Autodesk Inventor part; units mm, degrees
ref_plane "b1_XY" through (0, 7.8994, 0) normal (1, 0, 0) x (0, 0, -1)
ref_plane "b1_YZ" through (0, 7.8994, 0) normal (0, 0, -1) x (0, 1, 0)
ref_plane "b1_ZX" through (0, 7.8994, 0) normal (0, 1, 0) x (1, 0, 0)
sketch "Sketch_1" plane through (0, 0, 0) normal (0, 0, 1) x (1, 0, 0)
  line L0 (18.1102, 0) -> (0, 0)
  line L1 (0, 0) -> (0, 10.8585)
  line L2 (0, 10.8585) -> (18.1102, 10.8585)
  line L3 (18.1102, 10.8585) -> (18.1102, 0)
  line L4 (18.1102, 0) -> (0, 0)
revolve "Revolution1" add sketch "Sketch_1" angle 360 about axis through (18.1102, 0, 0) along (1, 0, 0)
sketch "Sketch_2" plane through (0, 0, 0) normal (0, 0, 1) x (1, 0, 0)
  line L0 (0, 0) -> (-12.7508, 0)
  line L1 (-12.7508, 0) -> (-12.7508, 7.098)
  line L2 (-12.7508, 7.098) -> (-11.9113, 7.9375)
  line L3 (-11.9113, 7.9375) -> (0, 7.9375)
  line L4 (0, 7.9375) -> (0, 0)
  line L5 (0, 0) -> (-12.7508, 0)
revolve "Revolution2" add sketch "Sketch_2" angle 360 about axis through (0, 0, 0) along (1, 0, 0)
thread "Thread1"
sketch "Sketch_6" plane through (0, 0, 0) normal (0, 0, 1) x (1, 0, 0)
  line L0 (27.7622, 0) -> (18.1102, 0)
  line L1 (18.1102, 0) -> (18.1102, 10.3505)
  line L2 (18.1102, 10.3505) -> (21.4122, 10.3505)
  line L3 (21.4122, 10.3505) -> (21.4122, 8.9027)
  line L4 (21.4122, 8.9027) -> (22.3266, 8.9027)
  line L5 (22.3266, 8.9027) -> (23.0505, 9.6266)
  line L6 (23.0505, 9.6266) -> (27.0002, 9.6266)
  line L7 (27.0002, 9.6266) -> (27.7622, 8.8646)
  line L8 (27.7622, 8.8646) -> (27.7622, 0)
  line L9 (27.7622, 0) -> (18.1102, 0)
revolve "Revolution3" add sketch "Sketch_6" angle 360 about axis through (27.7622, 0, 0) along (1, 0, 0)
sketch "Sketch_7" plane through (0, 0, 0) normal (1, 0, 0) x (0, 1, 0)
  circle A0 centre (0, 0) radius 3.175
extrude "Extrusion1" cut sketch "Sketch_7" along normal mid plane 111.0488
sketch "Sketch_8" plane through (11.8872, 0, 0) normal (0, 0, 1) x (0, -1, 0)
  line L0 (0, 0) -> (-11.7085, 0)
  line L1 (-11.7085, 0) -> (-11.7085, 6.4547)
  line L2 (-11.7085, 6.4547) -> (-10.0692, 4.8153)
  line L3 (-10.0692, 4.8153) -> (0, 4.501)
  line L4 (0, 4.501) -> (0, 0)
  line L5 (0, 0) -> (-11.7085, 0)
revolve "Revolution4" cut sketch "Sketch_8" angle 360 about axis through (11.8872, 0, 0) along (0, -1, 0)
sketch "Sketch_29" plane through (0, 0, 0) normal (0, 0, 1) x (1, 0, 0)
  line L0 (0, 0) -> (-4.6228, 0)
  line L1 (-4.6228, 9.8994) -> (-4.6228, 7.9375)
  line L2 (-4.6228, 7.9375) -> (-3.7284, 7.0431)
  arc A0 (-3.7284, 7.0431) -> (-3.1896, 6.8199) centre (-3.1896, 7.5819) ccw
  line L3 (-3.1896, 6.8199) -> (-2.7567, 6.8199)
  arc A1 (-2.7567, 6.8199) -> (-2.0828, 7.2263) centre (-2.7567, 7.5819) ccw
  line L4 (-2.0828, 7.2263) -> (-2.0828, 7.8994)
  line L5 (-2.0828, 7.8994) -> (0, 7.8994)
  line L6 (0, 7.8994) -> (0, 9.8994)
  line L7 (0, 9.8994) -> (-4.6228, 9.8994)
revolve "Revolution5" cut sketch "Sketch_29" angle 360 about axis through (0, 0, 0) along (1, 0, 0)
ref_plane "b1_XY" through (0, 7.8994, 0) normal (1, 0, 0) x (0, 0, -1)
ref_plane "b1_YZ" through (0, 7.8994, 0) normal (0, 0, -1) x (0, 1, 0)
ref_plane "b1_ZX" through (0, 7.8994, 0) normal (0, 1, 0) x (1, 0, 0)
ref_plane "b2_XY" through (0, -7.8994, 0) normal (1, 0, 0) x (0, 0, -1)
ref_plane "b2_YZ" through (0, -7.8994, 0) normal (0, 0, -1) x (0, 1, 0)
ref_plane "b2_ZX" through (0, -7.8994, 0) normal (0, 1, 0) x (1, 0, 0)
ref_plane "cl1_XY" through (0, 0, 0) normal (0, 0, 1) x (1, 0, 0)
ref_plane "cl1_YZ" through (0, 0, 0) normal (1, 0, 0) x (0, 1, 0)
ref_plane "cl1_ZX" through (0, 0, 0) normal (0, 1, 0) x (0, 0, 1)
ref_plane "cl2_XY" through (-2.0828, 0, 0) normal (0, 0, 1) x (1, 0, 0)
ref_plane "cl2_YZ" through (-2.0828, 0, 0) normal (1, 0, 0) x (0, 1, 0)
ref_plane "cl2_ZX" through (-2.0828, 0, 0) normal (0, 1, 0) x (0, 0, 1)
ref_plane "ee_XY" through (11.8872, 10.8585, 0) normal (1, 0, 0) x (0, -1, 0)
ref_plane "ee_YZ" through (11.8872, 10.8585, 0) normal (0, -1, 0) x (0, 0, -1)
ref_plane "ee_ZX" through (11.8872, 10.8585, 0) normal (0, 0, -1) x (1, 0, 0)
ref_plane "od1_XY" through (0, 0, 10.8585) normal (1, 0, 0) x (0, 0, -1)
ref_plane "od1_YZ" through (0, 0, 10.8585) normal (0, 0, -1) x (0, 1, 0)
ref_plane "od1_ZX" through (0, 0, 10.8585) normal (0, 1, 0) x (1, 0, 0)
ref_plane "od2_XY" through (0, 0, -10.8585) normal (1, 0, 0) x (0, 0, -1)
ref_plane "od2_YZ" through (0, 0, -10.8585) normal (0, 0, -1) x (0, 1, 0)
ref_plane "od2_ZX" through (0, 0, -10.8585) normal (0, 1, 0) x (1, 0, 0)
ref_plane "od3_XY" through (0, 10.8585, 0) normal (1, 0, 0) x (0, 0, -1)
ref_plane "od3_YZ" through (0, 10.8585, 0) normal (0, 0, -1) x (0, 1, 0)
ref_plane "od3_ZX" through (0, 10.8585, 0) normal (0, 1, 0) x (1, 0, 0)
ref_plane "od4_XY" through (0, -10.8585, 0) normal (1, 0, 0) x (0, 0, -1)
ref_plane "od4_YZ" through (0, -10.8585, 0) normal (0, 0, -1) x (0, 1, 0)
ref_plane "od4_ZX" through (0, -10.8585, 0) normal (0, 1, 0) x (1, 0, 0)
ref_plane "to_body_XY" through (21.4122, 0, 0) normal (1, 0, 0) x (0, 0, -1)
ref_plane "to_body_YZ" through (21.4122, 0, 0) normal (0, 0, -1) x (0, 1, 0)
ref_plane "to_body_ZX" through (21.4122, 0, 0) normal (0, 1, 0) x (1, 0, 0)
ref_plane "to_dummy_XY" through (0, 0, 0) normal (1, 0, 0) x (0, 0, -1)
ref_plane "to_dummy_YZ" through (0, 0, 0) normal (0, 0, -1) x (0, 1, 0)
ref_plane "to_dummy_ZX" through (0, 0, 0) normal (0, 1, 0) x (1, 0, 0)
ref_plane "to_nut_XY" through (-12.7508, 0, 0) normal (1, 0, 0) x (0, 0, -1)
ref_plane "to_nut_YZ" through (-12.7508, 0, 0) normal (0, 0, -1) x (0, 1, 0)
ref_plane "to_nut_ZX" through (-12.7508, 0, 0) normal (0, 1, 0) x (1, 0, 0)
ref_plane "to_stroke_adjuster_XY" through (27.7622, 0, 0) normal (1, 0, 0) x (0, 0, -1)
ref_plane "to_stroke_adjuster_YZ" through (27.7622, 0, 0) normal (0, 0, -1) x (0, 1, 0)
ref_plane "to_stroke_adjuster_ZX" through (27.7622, 0, 0) normal (0, 1, 0) x (1, 0, 0)
properties part number "0.75DXP-H_SRS1"
The model under review builds one solid part; all positions refer to its coordinate system, in mm. A direction names the side the tool comes from. Coordinates: 2 decimals unless noted, no trailing zeros. Write each loop counter-clockwise with the first axis right and the second up, starting at its lowest first coordinate (ties: lowest second). Pieces come first, ordered by that corner, then holes. Notation, with made-up numbers: M 32,61.25 L 80,61.25 A22 ccw 80,94.25 Z; hole C -30,72.5 d9. An arc over 180 degrees is marked long. Put each result on its own line as item: value.
1) Add section B-B on z = 0. State how many separate pieces and enclosed holes the cut face has, then the cut area to 3 significant figures.
Computed:
separate pieces: 3
enclosed holes: 0
area: 448 mm2
2) Add section A-A on x = 23.5. Give the boundary of the cut face in (y, z) (3 decimals).
Computed:
outline: C 0,0 d19.253; hole C 0,0 d6.35
3) Wall thickness on probe 1 along Z at (x, y) = (19.5, 0) (1 decimal); probe 2 along Z at (x, y) = (-3.5, -1.5); probe 3 along X at (y, z) = (4.25, -7.25): over which ranges is each line inside the solid? List them lowest first. Write a range as [from, to].
Computed:
probe 1: z = [-10.4, -3.2], [3.2, 10.4]
probe 2: z = [-6.72, -2.8], [2.8, 6.72]
probe 3: x = [0, 27.76]
4) For faces 1 (the conical face through (16.84, 10.21, 0.07)), 2 (the flat face through (27.762, 4, 0)), 3 (the cylindrical face through (9.182, -10.848, 0.477)), 4 (the cylindrical face through (19.78, -8.21, -6.3)), 5 (the cylindrical face through (21.876, 8.492, 2.674)), list the 3-axis set-ups (+Z, -Z, +X, -X, +Y, -Y) from which the entire face can be reached by the end or side of a thin tool; tool diameter is ignored.
Computed:
face 1: +Y
face 2: +Z, -Z, +X, +Y, -Y
face 3: +X, -X
face 4: +X
face 5: none
5) Clearance check with flat-ended pins moving along their axes: pin 1 Ø0.7 at (x, z) = (11, 4) entering from +Y; pin 2 Ø2 at (x, y) = (2, -5) entering from -Z; pin 3 Ø1.5 at (x, y) = (-8.5, -8) entering from -Z. State where each tip first meets the part, or that it passes through.
Computed:
pin 1: stops at y = 0
pin 2: stops at z = -10.09
pin 3: stops at z = -3.23
6) Draft analysis for pull direction X (two halves, no side actions). For faces 6 (the cylindrical face through (25.05, -7.64, -5.86)), 7 (the flat face through (-12.751, 3.1, -1.5)), 8 (the flat face through (12, 0, 4)), state which applies: released by +X, released by -X, zero draft, split by the parting line, or undercut.
Computed:
face 6: zero draft
face 7: released by -X
face 8: undercut
7) Add section C-C on x = -1. Give the boundary of the cut face in (y, z) (3 decimals).
Computed:
outline: C 0,0 d15.799; hole C 0,0 d6.35
